Read the model definition and answer for the solid it produces. Units are mm, in the model's axes. A direction names the side the tool comes from. Coordinates: 2 decimals unless noted, no trailing zeros. Order: outer loops, then holes, each group sorted by start corner. A loop starts at its lowest first (then second) coordinate and runs counter-clockwise, first axis right, second up. Notation, with made-up numbers: M 16,73.25 L 42,73.25 A19 ccw 42,88.25 Z; hole C -22.75,8.25 d5. An arc over 180 degrees is marked long. Use a Markdown table: item, result. Add a question column.
1) Each of these flat-tipped pins is pushed along its axis until it touches: pin 1 Ø0.8 at (y, z) = (4, -1) entering from -X; pin 2 Ø0.7 at (x, z) = (1, 0.5) entering from +Y. Where does it stop, or does it pass through?
2) Find section A-A on x = 0.95. Write down the section's boundary in (y, z), plus the area to 3 significant figures.
3) The mould has two halves that part along Y. Classify faces 3 (the face through (1.8, -5, 0)), 4 (the face through (1, -4.167, 0)), 5 (the face through (1.65, -1, -1)): released by +Y, released by -Y, zero draft, split by the parting line, or undercut.
4) Find section B-B on y = 0. Write down the section's boundary in (x, z), plus the area to 3 significant figures.
5) For faces 1 (the face through (0, -1, 0)), 2 (the face through (1.65, -5, 0)), determine the directions among +Z, -Z, +X, -X, +Y, -Y from which every point of the face is accessible in a straight line to the end or side of a thin tool.
6) Find the intervals of material crossed by probe 1 along X at (y, z) = (3.25, 1.25); probe 2 along X at (y, z) = (2.5, 0.5); probe 3 along Y at (x, z) = (1, 2.75), in increasing order. Write a range as [from, to].
from build123d import *

# Parameters (mm, degrees)
F1_DEPTH      = 1.5
F1_DEPTH_BACK = 1.5
F4_DEPTH      = 2
F4_DEPTH_BACK = 2
F5_R          = 1.99999


# Not quite as in the source:
# - a fillet or chamfer is up to 0.001 mm smaller than in the source, because OpenCascade refuses the exact size


with BuildPart() as f1:
    # F0 (on Top) → F1 (new body, two sides)
    with BuildSketch(Plane.XY) as f1_sk:
        with BuildLine():
            Line((0.15, 1.5), (0, 1.5))
            Line((0, 1.5), (0, 0))
            Line((0, 0), (0, -4))
            ThreePointArc((0, -4), (0.0487994019, -4.1178121778), (0.1666115796, -4.1666115796))
            Line((0.1666115796, -4.1666115796), (1.6031347549, -4.1666115796))
            ThreePointArc((1.6031347549, -4.1666115796), (1.6362734875, -4.1803380921), (1.65, -4.2134768248))
            Line((1.65, -4.2134768248), (1.65, -5.5134768248))
            Line((1.65, -5.5134768248), (1.8, -5.5134768248))
            Line((1.8, -5.5134768248), (1.8, -4.1666115796))
            ThreePointArc((1.8, -4.1666115796), (1.7560660172, -4.0605455625), (1.65, -4.0166115796))
            Line((1.65, -4.0166115796), (0.1968652451, -4.0166115796))
            ThreePointArc((0.1968652451, -4.0166115796), (0.1637265125, -4.0028850671), (0.15, -3.9697463345))
            Line((0.15, -3.9697463345), (0.15, 0))
            Line((0.15, 0), (0.15, 1.5))
        make_face()
    extrude(amount=F1_DEPTH)
    extrude(f1_sk.sketch, amount=-F1_DEPTH_BACK)

    # F0 (on Top) → F2 (revolve)
    with BuildSketch(Plane.XY):
        with BuildLine():
            Line((0.15, 2.6), (0.15, 1.5))
            Line((0.15, 1.5), (0.15, 0))
            Line((0.15, 0), (0.3, 0))
            Line((0.3, 0), (0.3, 2.7))
            Line((0.3, 2.7), (0.25, 2.7))
            ThreePointArc((0.25, 2.7), (0.1792893219, 2.6707106781), (0.15, 2.6))
        make_face()
    revolve(axis=Axis((0.225, 0, 0), (-1, 0, 0)))

    # F0 (on Top) → F3 (revolve)
    with BuildSketch(Plane.XY):
        with BuildLine():
            Line((0.3, 2.7), (0.3, 0))
            Line((0.3, 0), (1.65, 0))
            Line((1.65, 0), (1.65, 3.4))
            Line((1.65, 3.4), (0.7, 3.4))
            ThreePointArc((0.7, 3.4), (0.4171572875, 3.2828427125), (0.3, 3))
            Line((0.3, 3), (0.3, 2.7))
        make_face()
    revolve(axis=Axis((0.975, 0, 0), (-1, 0, 0)))

    # F0 (on Top) → F4 (join, two sides)
    with BuildSketch(Plane.XY) as f4_sk:
        Polygon((1.65, 3.4), (1.65, 0), (1.65, -1), (1.8, -1), (1.8, 5.5), (1.65, 5.5), align=None)
    extrude(amount=F4_DEPTH)
    extrude(f4_sk.sketch, amount=-F4_DEPTH_BACK)

    # F5 (radius 2 in the source; OpenCascade refuses exactly that, so slightly less here)
    f5_edges = [f1.edges().sort_by_distance(p)[0] for p in [
        (1.725, -1, -2),
        (1.725, -1, 2),
    ]]
    fillet(f5_edges, radius=F5_R)


solid = f1.part
Check result:
| question | item | result |
|---|---|---|
| 1 | pin 1 | stops at x = 1.65 |
| 1 | pin 2 | stops at y = 3.4 |
| 2 | outline | M -4.17,-1.5 L -4.02,-1.5 L -4.02,1.5 L -4.17,1.5 Z; C 0,0 d6.8 |
| 2 | area | 36.8 mm2 |
| 3 | face 3 | zero draft |
| 3 | face 4 | released by -Y |
| 3 | face 5 | undercut |
| 4 | outline | M 0,-1.5 L 0.15,-1.5 L 0.15,-2.6 A0.1 ccw 0.25,-2.7 L 0.3,-2.7 L 0.3,-3 A0.4 ccw 0.7,-3.4 L 1.65,-3.4 L 1.65,-1.73 L 1.8,-1.73 L 1.8,1.73 L 1.65,1.73 L 1.65,3.4 L 0.7,3.4 A0.4 ccw 0.3,3 L 0.3,2.7 L 0.25,2.7 A0.1 ccw 0.15,2.6 L 0.15,1.5 L 0,1.5 Z |
| 4 | area | 10.9 mm2 |
| 5 | face 1 | +Z, -Z, -X, +Y, -Y |
| 5 | face 2 | +Z, -Z, -X, -Y |
| 6 | probe 1 | x = [1.65, 1.8] |
| 6 | probe 2 | x = [0.15, 1.8] |
| 6 | probe 3 | y = [-2, 2] |
